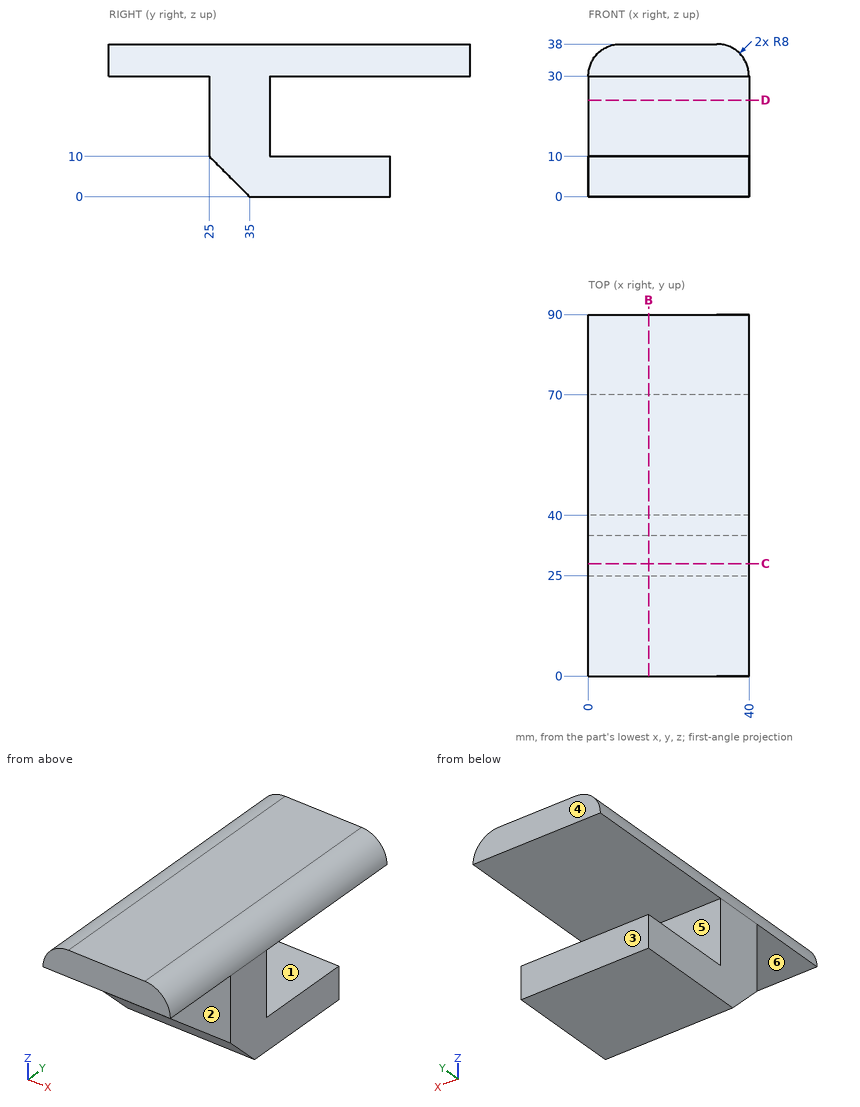
Print and shaded views of the part. All mm, measured from the part's lowest x, y and z. A direction names the side the tool comes from. Round coordinates to 2 decimals unless told otherwise and drop trailing zeros. Write each loop counter-clockwise with the first axis right and the second up, starting at its lowest first coordinate (ties: lowest second). Pieces come first, ordered by that corner, then holes. Notation, with made-up numbers: (-28.75, 10) - (20.25, 10) arc R17 ccw to (20.25, 27) - close; hole circle Ø8 at (24.5, 28). An arc over 180 degrees is marked (long way). One line per item, written item: value.
(1) Two-plate mould, pull along Z, no slides. Class the marked faces 4, 5 and 6: pulls with the +Z half, pulls with the -Z half, needs draft (parallel to the pull), parting line crosses it, or undercut.
Values follow:
face 4: needs draft
face 5: undercut
face 6: pulls with the -Z half
(2) Cut at B-B, the plane x = 15. Give the cut face in (y, z), plus the area to 3 significant figures.
Values follow:
outline: (0, 30) - (25, 30) - (25, 10) - (35, 0) - (70, 0) - (70, 10) - (40, 10) - (40, 30) - (90, 30) - (90, 38) - (0, 38) - close
area: 1,420 mm²
(3) Cut at D-D, the plane z = 24. Give the cut face in (x, y).
Values follow:
outline: (0, 25) - (40, 25) - (40, 40) - (0, 40) - close
(4) Drop flat-ended pins along their axis: P1, Ø16, axis at x = 27, z = 20, coming from the -Y side; P2, Ø1, axis at x = 5.5, z = 16.5, coming from the +Y side; P3, Ø7.5, axis at x = 25.5, y = 7, coming from the -Z side. Give the stop position or say it passes through.
Values follow:
P1: stops at y = 25
P2: stops at y = 40
P3: stops at z = 30
(5) Cut at C-C, the plane y = 28. Give the cut face in (x, z), plus the area to 3 significant figures.
Values follow:
outline: (0, 7) - (40, 7) - (40, 30) arc R8 ccw to (32, 38) - (8, 38) arc R8 ccw to (0, 30) - close
area: 1,210 mm²
(6) Wall check: probe 1 along Z at (x, y) = (31, 55); probe 2 along Y at (x, z) = (4.5, 14); probe 3 along Z at (x, y) = (23, 19.5). Give the ranges that are in metal, low to high.
Values follow:
probe 1: z = 0 to 10, 30 to 38
probe 2: y = 25 to 40
probe 3: z = 30 to 38
(7) 3-axis set-ups, long thin cutter, end or side, ignore diameter. For the marked faces 1, 2 and 3: which of +Z, -Z, +X, -X, +Y, -Y reach the whole face in a straight line?
Values follow:
face 1: +X, -X, +Y
face 2: -Z, +X, -X, -Y
face 3: -Z, +X, -X, +Y
